Verification items for the finished model (mm, model axes). A direction names the side the tool comes from. Round coordinates to 2 decimals unless told otherwise and drop trailing zeros. Write each loop counter-clockwise with the first axis right and the second up, starting at its lowest first coordinate (ties: lowest second). Pieces come first, ordered by that corner, then holes.
Autodesk Inventor part; units mm, degrees
ref_plane "YZ Plane" through (0, 0, 0) normal (1, 0, 0) x (0, 1, 0)
ref_plane "XZ Plane" through (0, 0, 0) normal (0, 1, 0) x (-1, 0, 0)
ref_plane "XY Plane" through (0, 0, 0) normal (0, 0, 1) x (1, 0, 0)
sketch "TopProfile" plane through (0, 0, 0) normal (0, 0, 1) x (1, 0, 0)
  line L0 (0, 0) -> (66.675, 0)
  line L1 (66.675, 0) -> (66.675, 34.925)
  line L2 (66.675, 34.925) -> (0, 34.925)
  line L3 (0, 34.925) -> (0, 0)
  line L4 (1.5875, 30.5594) -> (65.0875, 30.5594)
  line L5 (65.0875, 30.5594) -> (65.0875, 4.3656)
  line L6 (65.0875, 4.3656) -> (1.5875, 4.3656)
  line L7 (1.5875, 4.3656) -> (1.5875, 30.5594)
  line L8 (25.4, 4.3656) -> (41.275, 4.3656)
  line L9 (41.275, 4.3656) -> (41.275, 2.7781)
  line L10 (41.275, 2.7781) -> (25.4, 2.7781)
  line L11 (25.4, 2.7781) -> (25.4, 4.3656)
  line L12 (4.3656, 27.7812) -> (62.3094, 27.7812)
  line L13 (62.3094, 27.7812) -> (62.3094, 11.9063)
  line L14 (62.3094, 11.9063) -> (4.3656, 11.9062)
  line L15 (4.3656, 11.9062) -> (4.3656, 27.7812)
  point P0 (33.3375, 4.3656)
  dimension "d0" = 66.675
  dimension "d1" = 34.925
  dimension "d2" = 26.1938
  dimension "d3" = 63.5
  dimension "d4" = 1.5875
  dimension "d5" = 1.6002
  dimension "d6" = 27.7812
  dimension "d7" = 15.875
  dimension "d8" = 4.3656
  dimension "d9" = 15.875
  dimension "d10" = 2.7781
  dimension "d11" = 2.7781
  dimension "d12" = 2.7781
extrude "BoardFeature" add sketch "TopProfile" against normal blind 0.7937 contours L3 L2 L1 L0 | L4 L5 L6 L7 | L6 L9 L10 L11 | L12 L13 L14 L15
extrude "ScreenFeature" add sketch "TopProfile" along normal blind 5.1594 contours L4 L5 L6 L7 | L6 L9 L10 L11
extrude "DisplayFeature" add sketch "TopProfile" along normal blind 4.572 contours L12 L13 L14 L15
fillet "BezelFilletsFeature" radius 0.254 4 edges at (4.3656, 27.7812, 4.8657) (62.3094, 27.7812, 4.8657) (62.3094, 11.9063, 4.8657) (4.3656, 11.9062, 4.8657)
fillet "BottomFilletsFeature" radius 1.524 2 edges at (25.4, 2.7781, 2.5797) (41.275, 2.7781, 2.5797)
sketch "MountHoles" plane through (0, 0, 0) normal (0, 0, 1) x (1, 0, 0)
  circle A0 centre (0.7937, 0.7937) radius 0.7937
  circle A1 centre (65.8813, 0.7937) radius 0.7937
  line L0 (0, 0) -> (66.675, 0) construction
  line L1 (0, 34.925) -> (0, 0) construction
  line L2 (66.675, 0) -> (66.675, 34.925) construction
  circle A2 centre (0.7937, 34.1313) radius 0.7937
  circle A3 centre (65.8812, 34.1313) radius 0.7937
  line L3 (66.675, 34.925) -> (0, 34.925) construction
  dimension "d21" = 1.5875
  dimension "d32" = 65.0875
hole "MountHolesFeature" at (0.7937, 0.7937, 0) at (0.7937, 34.1313, 0) at (65.8812, 34.1313, 0) at (65.8813, 0.7937, 0) direction (0, 0, -1) diameter 1.27 end through all
equation "\"d11\" = d10"
equation "\"d12\" = d10"
properties part number "oscilloscope-screen"
Q1. Sectioned sample at B-B (y = 20.5). Enter the section's corners in (x, z) (1 decimal), plus the area to 3 significant figures.
Recorded:
outline: (0, -0.8) - (66.7, -0.8) - (66.7, 0) - (65.1, 0) - (65.1, 5.2) - (62.3, 5.2) - (62.3, 4.6) - (4.4, 4.6) - (4.4, 5.2) - (1.6, 5.2) - (1.6, 0) - (0, 0) - close
area: 347 mm2
Q2. Release check for a two-part mould opening along Y. For faces 5 (the cylindrical face through (66.5, 0.93, -0.4)), 6 (the flat face through (33, 11, 5.159)), 7 (the cylindrical face through (25.83, 3.24, 2.62)) record: released by +Y, released by -Y, zero draft, split by the parting line, or undercut.
Recorded:
face 5: undercut
face 6: zero draft
face 7: released by -Y
Q3. Sectioned sample at C-C (x = 10.5). Enter the section's corners in (y, z) (3 decimals).
Recorded:
outline: (0, -0.794) - (34.925, -0.794) - (34.925, 0) - (30.559, 0) - (30.559, 5.159) - (27.781, 5.159) - (27.781, 4.572) - (11.906, 4.572) - (11.906, 5.159) - (4.366, 5.159) - (4.366, 0) - (0, 0) - close
Q4. Material ranges on line 1 along Y through (x, z) = (59.5, 4.9); line 2 along Y through (x, z) = (49, 2.65); line 3 along X through (y, z) = (6, 2.8), recorded low to high.
Recorded:
line 1: y = 4.37 to 11.91, 27.78 to 30.56
line 2: y = 4.37 to 30.56
line 3: x = 1.59 to 65.09
Q5. Depth check by flat-ended pin: P1, Ø2.5, axis at x = 14.5, z = 2, coming from the -Y side; P2, Ø6, axis at x = 42.5, y = 18.5, coming from the +Z side; P3, Ø1.7, axis at x = 0.79, y = 34.13, coming from the +Z side. Enter the tip coordinate at first touch or a pass-through.
Recorded:
P1: stops at y = 4.37
P2: stops at z = 4.57
P3: stops at z = 0
Q6. Tool access check on faces 1 (the flat face through (33, 20, 4.572)), 2 (the flat face through (33, 2.778, 3)), 3 (the flat face through (14, 4.366, 3)), 4 (the cylindrical face through (40.817, 3.213, 2.616)). Record the directions out of +Z, -Z, +X, -X, +Y, -Y that give a thin tool (end or side, any length) a straight path to the whole face; none if there is none.
Recorded:
face 1: +Z
face 2: +Z, +X, -X, -Y
face 3: +Z, -X, -Y
face 4: +Z, +X, -Y
Q7. Sectioned sample at D-D (y = 31.5). Enter the section's corners in (x, z) (3 decimals).
Recorded:
outline: (0, -0.794) - (66.675, -0.794) - (66.675, 0) - (0, 0) - close
